Read the model definition and answer for the solid it produces. Units are mm, in the model's axes. Coordinates: 2 decimals unless noted, no trailing zeros. Order: outer loops, then holes, each group sorted by start corner. A loop starts at its lowest first (then second) coordinate and runs counter-clockwise, first axis right, second up.
```python
from build123d import *

# Parameters (mm, degrees)
SKETCH1_R           = 111.125
SKETCH1_R_2         = 3.96875
SKETCH1_R_3         = 9.75
BOSS_EXTRUDE1_DEPTH = 1.5875


with BuildPart() as part:
    # Sketch1 → Boss-Extrude1 (new body)
    with BuildSketch(Plane(origin=(0, 0, 0), x_dir=(1, 0, 0), z_dir=(0, 1, 0))):
        with Locations((0, 2.067110037)):
            Circle(SKETCH1_R)
        with Locations((4.071636725, 23.915963539)):
            Circle(SKETCH1_R_2, mode=Mode.SUBTRACT)
        with Locations((-20.957480539, -5.331175876)):
            Circle(SKETCH1_R_2, mode=Mode.SUBTRACT)
        with Locations((16.885843815, -12.383457553)):
            Circle(SKETCH1_R_2, mode=Mode.SUBTRACT)
        with Locations((-44.897615706, 23.149190197)):
            Circle(SKETCH1_R_3, mode=Mode.SUBTRACT)
        with Locations((-49.477634519, -1.427697882)):
            Circle(SKETCH1_R_3, mode=Mode.SUBTRACT)
        with Locations((-68.471834536, 14.827158799)):
            Circle(SKETCH1_R_3, mode=Mode.SUBTRACT)
        with Locations((68.471834536, -10.692938726)):
            Circle(SKETCH1_R_3, mode=Mode.SUBTRACT)
        with Locations((44.897615706, -19.014970124)):
            Circle(SKETCH1_R_3, mode=Mode.SUBTRACT)
        with Locations((49.477634519, 5.561917956)):
            Circle(SKETCH1_R_3, mode=Mode.SUBTRACT)
        Polygon((3.519990025, -41.816901652), (5.443597926, -31.494608658), (-17.167139107, -27.28099135), (-19.090747008, -37.603284344), align=None, mode=Mode.SUBTRACT)
        with BuildLine():
            ThreePointArc((90.719240331, 17.809570412), (16.868209288, 92.583788834), (-78.959268715, 49.429959498))
            ThreePointArc((-78.959268715, 49.429959498), (-78.745756198, 42.56506275), (-72.411496849, 39.909963234))
            ThreePointArc((-72.411496849, 39.909963234), (6.979948671, 39.52228747), (81.18188186, 11.287113924))
            ThreePointArc((81.18188186, 11.287113924), (88.04732163, 11.482387358), (90.719240331, 17.809570412))
        make_face(mode=Mode.SUBTRACT)
        with BuildLine():
            ThreePointArc((-34.133508794, -73.846482708), (-46.481955973, -29.811909239), (-83.112792301, -2.431083134))
            ThreePointArc((-83.112792301, -2.431083134), (-89.116651342, -3.572720267), (-91.376738817, -9.250894562))
            ThreePointArc((-91.376738817, -9.250894562), (-75.932582562, -50.010222177), (-43.472216603, -79.099213082))
            ThreePointArc((-43.472216603, -79.099213082), (-37.361105633, -79.036114425), (-34.133508794, -73.846482708))
        make_face(mode=Mode.SUBTRACT)
        with BuildLine():
            ThreePointArc((4.498193171, -81.045682265), (31.879019276, -44.414845936), (75.913592744, -32.066398757))
            ThreePointArc((75.913592744, -32.066398757), (81.103224462, -35.293995597), (81.166323119, -41.405106566))
            ThreePointArc((81.166323119, -41.405106566), (52.077332214, -73.865472525), (11.318004599, -89.309628781))
            ThreePointArc((11.318004599, -89.309628781), (5.639830304, -87.049541305), (4.498193171, -81.045682265))
        make_face(mode=Mode.SUBTRACT)
    extrude(amount=BOSS_EXTRUDE1_DEPTH)


solid = part.part
```
1) Determine the mould class of faces 1 (the cylindrical face through (-14.466, 0.783, -112.246)), 2 (the flat face through (-2, 0, 21)), 3 (the cylindrical face through (5.881, 0.783, -39.724)) for opening direction Z: pulls with the +Z half, pulls with the -Z half, needs draft (parallel to the pull), parting line crosses it, or undercut.
A:
face 1: parting line crosses it
face 2: needs draft
face 3: undercut
2) A flat-ended cylindrical pin translates along its axis: pin 1 Ø10 at (x, z) = (10.5, 58.5) entering from -Y. Find the tip coordinate at first contact, or state that the pin passes through.
A:
pin 1: stops at y = 0
3) A cutting plane is placed at D-D, the plane y = 0.6. State how many separate pieces and enclosed holes the cut face has, and give its area (3 significant figures).
A:
separate pieces: 1
enclosed holes: 13
area: 24,300 mm2
4) Straight lines are drawn through the part: line 1 (Z direction, x = 19, y = 0.45); line 2 (X direction, y = 1.55, z = -27); line 3 (Z direction, x = 2.5, y = 1). For each, find the intervals that lie inside material, in ascending order.
A:
line 1: z = -111.56 to -92.16, -36.94 to 9.02, 15.74 to 55.76, 88.03 to 107.42
line 2: x = -108.29 to -53.85, -35.94 to 1.57, 6.57 to 49.78, 88.63 to 108.29
line 3: z = -113.16 to -94.11, -40.31 to -27.56, -20.27 to 30.95, 41.63 to 109.03
5) A cutting plane is placed at B-B, the plane z = -76. Determine the outline of the cut face in (x, y).
A:
outline: (-82.96, 0) - (-54.88, 0) - (-54.88, 1.59) - (-82.96, 1.59) - close; (54.88, 0) - (82.96, 0) - (82.96, 1.59) - (54.88, 1.59) - close
6) A cutting plane is placed at A-A, the plane x = -6. Determine the outline of the cut face in (y, z), and give its area (3 significant figures).
A:
outline: (0, -113.03) - (1.59, -113.03) - (1.59, -93.95) - (0, -93.95) - close; (0, -41.55) - (1.59, -41.55) - (1.59, 29.36) - (0, 29.36) - close; (0, 40.04) - (1.59, 40.04) - (1.59, 108.9) - (0, 108.9) - close
area: 252 mm2
7) A cutting plane is placed at C-C, the plane x = 86.5. Determine the outline of the cut face in (y, z).
A:
outline: (0, -71.83) - (1.59, -71.83) - (1.59, -33.62) - (0, -33.62) - close; (0, -10.71) - (1.59, -10.71) - (1.59, 67.69) - (0, 67.69) - close
